Part model, mm, in its own coordinate system. Face numbers are marked on the shaded views. A direction names the side the tool comes from. Coordinates: 2 decimals unless noted, no trailing zeros. Order: outer loops, then holes, each group sorted by start corner. A loop starts at its lowest first (then second) coordinate and runs counter-clockwise, first axis right, second up.
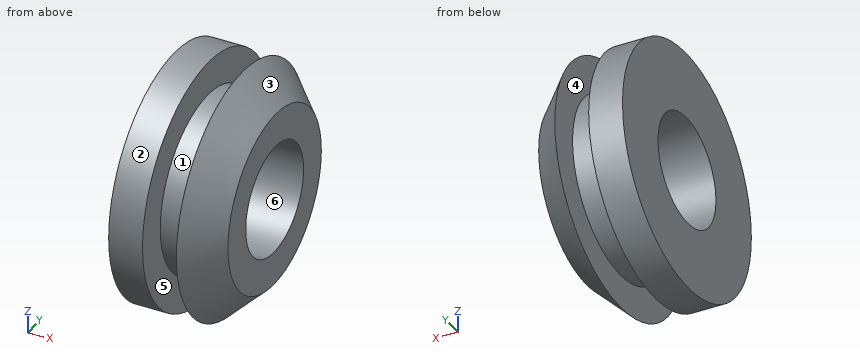
Autodesk Inventor part; units mm, degrees
ref_plane "作業平面1" through (0.5, 0, 0) normal (1, 0, 0) x (0, 0, -1)
ref_plane "YZ Plane" through (0, 0, 0) normal (1, 0, 0) x (0, 1, 0)
ref_plane "XZ Plane" through (0, 0, 0) normal (0, 1, 0) x (-1, 0, 0)
sketch "スケッチ1" plane through (0, 0, 0) normal (1, 0, 0) x (0, 1, 0)
  circle A0 centre (0, 0) radius 3.635
  circle A1 centre (0, 0) radius 1.635
  circle A2 centre (0, 0) radius 2.635
  dimension "d0" = 3.27
  dimension "d1" = 2
  dimension "d7" = 1
extrude "押し出し1" add sketch "スケッチ1" along normal mid plane 3 contours A0 | A2
ref_plane "作業平面1" through (0.5, 0, 0) normal (1, 0, 0) x (0, 0, -1)
extrude "押し出し3" cut sketch "スケッチ1" against normal blind 1 from surface at 0.5 contours A0
chamfer "面取り3" distance 1 angle 45 1 edges at (1.5, -3.635, 0)
properties part number "spacer_Φ3.2_1"
Q1. Cut at C-C on x = 0.2. Write the cut outline in (y, z) (3 decimals), and give its area (3 significant figures).
Results list:
outline: circle Ø5.27 at (0, 0); hole circle Ø3.27 at (0, 0)
area: 13.4 mm2
Q2. Wall check: line 1 along Z through (x, y) = (-0.1, 0) (3 decimals); line 2 along Y through (x, z) = (-1.1, 0.5); line 3 along Y through (x, z) = (0.3, 1.5). Give the ranges that are in metal, low to high.
Results list:
line 1: z = -2.635 to -1.635, 1.635 to 2.635
line 2: y = -3.6 to -1.56, 1.56 to 3.6
line 3: y = -2.17 to -0.65, 0.65 to 2.17
Q3. Mould opens along X. For the marked faces 1, 2, 3 and 4 say: pulls with the +X half, pulls with the -X half, needs draft (parallel to the pull), parting line crosses it, or undercut.
Results list:
face 1: undercut
face 2: needs draft
face 3: pulls with the +X half
face 4: undercut
Q4. Which spindle directions (+Z, -Z, +X, -X, +Y, -Y) get a long thin tool onto all of the face, cutting with end or side? Do the marked faces 5 and 6. Say none if no direction does.
Results list:
face 5: none
face 6: +X, -X
